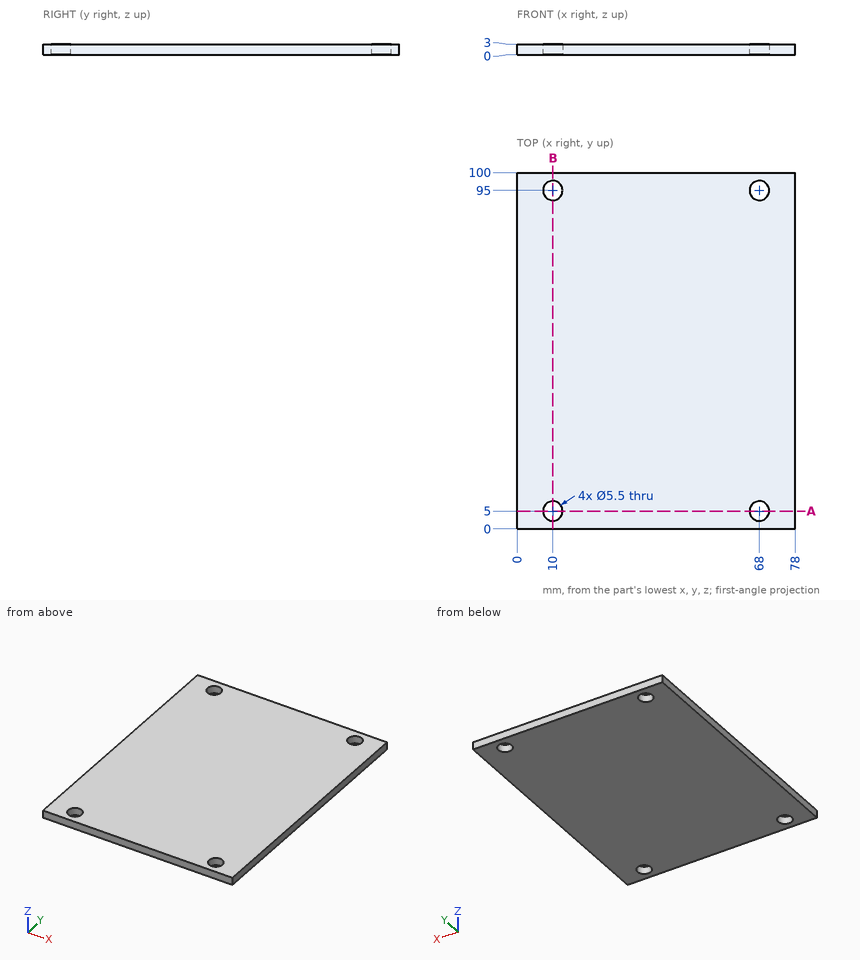
Geometry: see drawing. Coordinates: mm, zero at the bounding-box minimum. Round coordinates to 2 decimals unless told otherwise and drop trailing zeros. Loops run counter-clockwise (first coordinate to the right, second up) from the corner with the lowest first, then second, coordinate; pieces in that order, holes last. Notation, with made-up numbers: M 71,8 L 123,8 A14 ccw 123,23 Z; hole C 27,45 d9. An arc over 180 degrees is marked long. Use a Markdown table: item, result. Add a question column.
1. Ray query, line 1 along Y through (x, z) = (10, 1.7); line 2 along Y through (x, z) = (12.5, 0.65); line 3 along X through (y, z) = (7.5, 1.8). Return the intervals inside material, ascending. Write a range as [from, to].
2. Cut plane B-B, the plane x = 10. Output: boundary loops of the cut face in (y, z), and give its area (3 significant figures).
3. Cut plane A-A, the plane y = 5. Output: boundary loops of the cut face in (x, z).
Solution:
| question | item | result |
|---|---|---|
| 1 | line 1 | y = [0, 2.25], [7.75, 92.25], [97.75, 100] |
| 1 | line 2 | y = [0, 3.85], [6.15, 93.85], [96.15, 100] |
| 1 | line 3 | x = [0, 8.85], [11.15, 66.85], [69.15, 78] |
| 2 | outline | M 0,0 L 2.25,0 L 2.25,3 L 0,3 Z; M 7.75,0 L 92.25,0 L 92.25,3 L 7.75,3 Z; M 97.75,0 L 100,0 L 100,3 L 97.75,3 Z |
| 2 | area | 267 mm2 |
| 3 | outline | M 0,0 L 7.25,0 L 7.25,3 L 0,3 Z; M 12.75,0 L 65.25,0 L 65.25,3 L 12.75,3 Z; M 70.75,0 L 78,0 L 78,3 L 70.75,3 Z |
